from build123d import *

# Parameters (mm, degrees)
F0_W     = 30
F0_H     = 4.5
F1_DEPTH = 1.25
F3_DEPTH = 1.25


with BuildPart() as f1:
    # F0 (on Front) → F1 (new body)
    with BuildSketch(Plane.XZ):
        with Locations((15, 2.25)):
            Rectangle(F0_W, F0_H)
    extrude(amount=F1_DEPTH)

    # F2 (on face) → F3 (join)
    with BuildSketch(Plane.XZ.offset(1.25)):
        Polygon((0, 0), (0, 4.5), (0, 5.25), (-1, 5.25), (-1, -0.75), (0, -0.75), align=None)
        Polygon((30, 5.25), (30, 4.5), (30, 0), (30, -0.75), (31, -0.75), (31, 5.25), align=None)
    extrude(amount=-F3_DEPTH)


solid = f1.part
For this review, take the finished solid that the model builds, in its own axes (mm). A direction names the side the tool comes from. Give positions to 0.01 mm unless a question says otherwise; leave off trailing zeros. Order: outer loops, then holes, each group sorted by start corner. A loop starts at its lowest first (then second) coordinate and runs counter-clockwise, first axis right, second up. Notation, with made-up numbers: (75.25, -10) - (116.25, -10) arc R17 ccw to (116.25, 2) - close; hole circle Ø1 at (39.25, -36.5). An arc over 180 degrees is marked (long way). Answer as a JSON object with one key per item and string values. Group by question number.
Item 1: Take a section at A-A on y = -0.55. Give the boundary of the cut face in (x, z), and give its area (3 significant figures).
Item 2: Clearance check with a flat-ended pin moving along its axis: pin 1 Ø0.6 at (x, y) = (17, -0.5) entering from +Z. State where the tip first meets the part, or that it passes through.
Item 3: Machinability: for faces 1 (the flat face through (30.5, -0.6, 5.25)), 2 (the flat face through (15, -1, 0)), 3 (the flat face through (15, -1, 4.5)), which of the approach directions +Z, -Z, +X, -X, +Y, -Y give a long, thin tool a straight path to every point of the face, cutting with its end or side? Answer none if there is none.
Item 4: Take a section at B-B on x = 26.5. Give the boundary of the cut face in (y, z), and give its area (4 significant figures).
Item 5: Wall thickness on line 1 along X through (y, z) = (-0.85, -0.25); line 2 along Z through (x, y) = (10, -0.4): over which ranges is each line inside the solid? List them lowest first.
Reported:
{
 "1": {"outline": "(-1, -0.75) - (0, -0.75) - (0, 0) - (30, 0) - (30, -0.75) - (31, -0.75) - (31, 5.25) - (30, 5.25) - (30, 4.5) - (0, 4.5) - (0, 5.25) - (-1, 5.25) - close", "area": "147 mm^2"},
 "2": {"pin 1": "z = 4.5"},
 "3": {"face 1": "+Z, +X, -X, +Y, -Y", "face 2": "-Z, +Y, -Y", "face 3": "+Z, +Y, -Y"},
 "4": {"outline": "(-1.25, 0) - (0, 0) - (0, 4.5) - (-1.25, 4.5) - close", "area": "5.625 mm^2"},
 "5": {"line 1": "-1 to 0, 30 to 31", "line 2": "0 to 4.5"}
}
